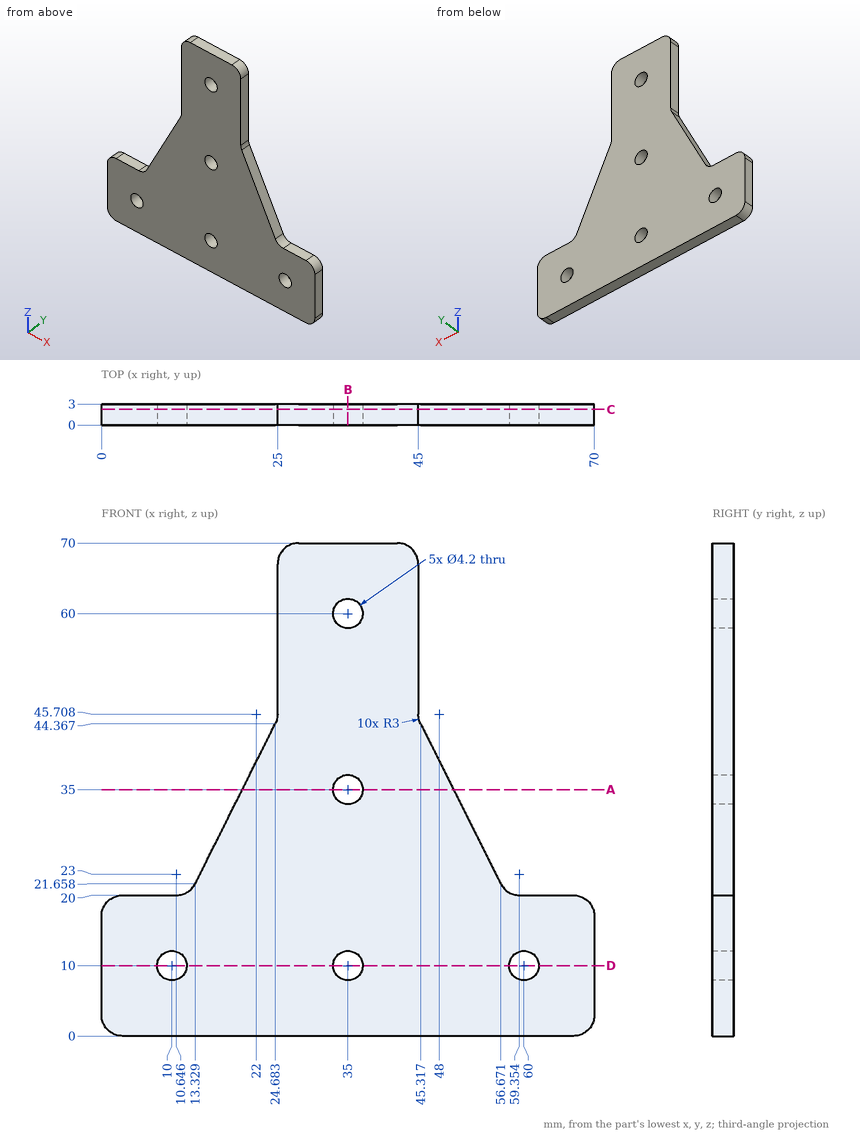
Part print with two shaded views. Sizes in mm from the minimum x, y, z corner. Coordinates: 2 decimals unless noted, no trailing zeros. Write each loop counter-clockwise with the first axis right and the second up, starting at its lowest first coordinate (ties: lowest second). Pieces come first, ordered by that corner, then holes. Notation, with made-up numbers: M -24.5,-27 L 14.5,-27 A24 cw 14.5,-14 Z; hole C 63,80.25 d1. An arc over 180 degrees is marked long. Return JSON: item names as keys, results as strings.
Item 1: Drop flat-ended pins along their axis: pin 1 Ø4 at (x, z) = (60, 10) entering from -Y; pin 2 Ø5 at (x, z) = (35, 60) entering from -Y; pin 3 Ø1.5 at (x, y) = (8.5, 1.5) entering from +Z; pin 4 Ø0.9 at (y, z) = (1.5, 55.5) entering from +X. Give the stop position or say it passes through.
Findings below:
{"pin 1": "passes through", "pin 2": "stops at y = 0", "pin 3": "stops at z = 20", "pin 4": "stops at x = 45"}
Item 2: Probe line 1 (X direction, y = 1.35, z = 10); line 2 (X direction, y = 2.6, z = 11) (1 decimal); line 3 (Z direction, x = 5.5, y = 1.75). List the from-to ranges inside material, lowest first. Write a range as from..to.
Findings below:
{"line 1": "x = 0..7.9, 12.1..32.9, 37.1..57.9, 62.1..70", "line 2": "x = 0..8.2, 11.8..33.2, 36.8..58.2, 61.8..70", "line 3": "z = 0..20"}
Item 3: Slice it at C-C, the plane y = 2.25. Write the cut outline in (x, z).
Findings below:
{"outline": "M 0,3 A3 ccw 3,0 L 67,0 A3 ccw 70,3 L 70,17 A3 ccw 67,20 L 59.35,20 A3 cw 56.67,21.66 L 45.32,44.37 A3 cw 45,45.71 L 45,67 A3 ccw 42,70 L 28,70 A3 ccw 25,67 L 25,45.71 A3 cw 24.68,44.37 L 13.33,21.66 A3 cw 10.65,20 L 3,20 A3 ccw 0,17 Z; hole C 10,10 d4.2; hole C 35,10 d4.2; hole C 35,35 d4.2; hole C 35,60 d4.2; hole C 60,10 d4.2"}
Item 4: Slice it at A-A, the plane z = 35. Write the cut outline in (x, y).
Findings below:
{"outline": "M 20,0 L 32.9,0 L 32.9,3 L 20,3 Z; M 37.1,0 L 50,0 L 50,3 L 37.1,3 Z"}
Item 5: Slice it at D-D, the plane z = 10. Write the cut outline in (x, y).
Findings below:
{"outline": "M 0,0 L 7.9,0 L 7.9,3 L 0,3 Z; M 12.1,0 L 32.9,0 L 32.9,3 L 12.1,3 Z; M 37.1,0 L 57.9,0 L 57.9,3 L 37.1,3 Z; M 62.1,0 L 70,0 L 70,3 L 62.1,3 Z"}
Item 6: Slice it at B-B, the plane x = 35. Write the cut outline in (y, z), and give its area (3 significant figures).
Findings below:
{"outline": "M 0,0 L 3,0 L 3,7.9 L 0,7.9 Z; M 0,12.1 L 3,12.1 L 3,32.9 L 0,32.9 Z; M 0,37.1 L 3,37.1 L 3,57.9 L 0,57.9 Z; M 0,62.1 L 3,62.1 L 3,70 L 0,70 Z", "area": "172 mm2"}
